Verification items for the finished model (mm, model axes). Give positions to 0.01 mm unless a question says otherwise; leave off trailing zeros. Order: outer loops, then holes, each group sorted by start corner. A loop starts at its lowest first (then second) coordinate and runs counter-clockwise, first axis right, second up.
from build123d import *

# Parameters (mm, degrees)
SKETCH2_R           = 1.5
CUT_EXTRUDE1_DEPTH  = 6
SKETCH2_3_R         = 3.5
SKETCH2_3_R_2       = 1.5
BOSS_EXTRUDE1_DEPTH = 10


with BuildPart() as part:
    # Sketch1 → Revolve1 (revolve)
    with BuildSketch(Plane.XY):
        with BuildLine():
            Line((0, 5), (0, -5))
            ThreePointArc((0, -5), (5, 0), (0, 5))
        make_face()
    revolve(axis=Axis((0, 5, 0), (0, -1, 0)))

    # Sketch2 → Cut-Extrude1 (cut, through all)
    with BuildSketch(Plane.XY):
        with Locations(Location((0, 0, 0), (0, 0, 180))):  # turned: the seam where the file's is
            Circle(SKETCH2_R)
    extrude(amount=CUT_EXTRUDE1_DEPTH, mode=Mode.SUBTRACT)

    # Sketch2_3 → Boss-Extrude1 (add)
    with BuildSketch(Plane.XY):
        with Locations(Location((0, 0, 0), (0, 0, 180))):  # turned: the seam where the file's is
            Circle(SKETCH2_3_R)
        Circle(SKETCH2_3_R_2, mode=Mode.SUBTRACT)
    extrude(amount=BOSS_EXTRUDE1_DEPTH)


solid = part.part
(1) Section check C-C, the plane x = 1.25. Enter the section's corners in (y, z).
Solved:
outline: (-3.27, 3.57) arc R4.84 ccw (long way) to (3.27, 3.57) - (3.27, 10) - (0.83, 10) - (0.83, 0) - (-0.83, 0) - (-0.83, 10) - (-3.27, 10) - close
(2) Section check A-A, the plane y = 0. Enter the section's corners in (x, z), then the cut area to 3 significant figures.
Solved:
outline: (-3.5, 3.57) arc R5 ccw (long way) to (3.5, 3.57) - (3.5, 10) - (1.5, 10) - (1.5, 0) - (-1.5, 0) - (-1.5, 10) - (-3.5, 10) - close
area: 86.7 mm2
(3) Section check D-D, the plane z = -1.75. Enter the section's corners in (x, y).
Solved:
outline: circle Ø9.37 at (0, 0)
(4) Release check for a two-part mould opening along Y. For faces 1 (the flat face through (0, 0, 0)), 2 (the flat face through (-2, 0, 10)), 3 (the cylindrical face through (-3.233, 1.341, 6.74)) record: pulls with the +Y half, pulls with the -Y half, needs draft (parallel to the pull), parting line crosses it, or undercut.
Solved:
face 1: undercut
face 2: needs draft
face 3: parting line crosses it
(5) Go/stop test with flat-tipped pins: pin 1 (3 mm diameter, centred on y = 0, z = 2, fed in from -X); pin 2 (3 mm diameter, centred on x = -3, z = -0.5, fed in from +Y); pin 3 (2.5 mm diameter, centred on x = 0.5, y = -0.5, fed in from +Z); pin 4 (4 mm diameter, centred on y = -3, z = 6, fed in from -X). Record where each tip stops, or that it passes through.
Solved:
pin 1: stops at x = -4.97
pin 2: stops at y = 4.76
pin 3: stops at z = 10
pin 4: stops at x = -3.35
(6) Section check B-B, the plane z = 7.75. Enter the section's corners in (x, y).
Solved:
outline: circle Ø7 at (0, 0); hole circle Ø3 at (0, 0)
(7) Scan lines: line 1 (Y direction, x = 0, z = 6.2); line 2 (Y direction, x = 0, z = 2.2); line 3 (Z direction, x = 3.25, y = 3). Record each from-to range of solid material in increasing order.
Solved:
line 1: y = -3.5 to -1.5, 1.5 to 3.5
line 2: y = -4.49 to -1.5, 1.5 to 4.49
line 3: z = -2.33 to 2.33
